Verification items for the finished model (mm, model axes). Face numbers are marked on the shaded views. A direction names the side the tool comes from. Give positions to 0.01 mm unless a question says otherwise; leave off trailing zeros. Loops run counter-clockwise (first coordinate to the right, second up) from the corner with the lowest first, then second, coordinate; pieces in that order, holes last. Notation, with made-up numbers: M 46,21.5 L 59,21.5 A24 ccw 59,33.5 Z; hole C -13.5,-4 d10. An arc over 180 degrees is marked long. Use CSV: the item, a comma, the result in double quotes.
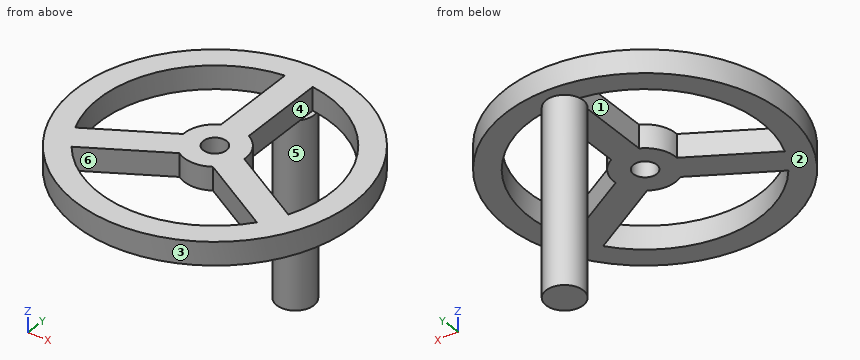
from build123d import *

# Parameters (mm, degrees)
SKETCH1_R           = 76.2
SKETCH1_R_2         = 63.5
SKETCH1_R_3         = 16.816105372
SKETCH1_R_4         = 6.35
BOSS_EXTRUDE1_DEPTH = 12.7
SKETCH2_R           = 10.16
BOSS_EXTRUDE2_DEPTH = 101.6


with BuildPart() as part:
    # Sketch1 → Boss-Extrude1 (new body)
    # profile 1 of 6: a face of its own
    with BuildSketch(Plane.XY):
        Circle(SKETCH1_R)
        Circle(SKETCH1_R_2, mode=Mode.SUBTRACT)
    # profile 2 of 6: a face of its own
    with BuildSketch(Plane.XY):
        with BuildLine():
            ThreePointArc((-7.62, 14.990563695), (-3.917811966, 16.353352845), (0, 16.816105372))
            Line((0, 16.816105372), (0, 63.5))
            ThreePointArc((0, 63.5), (-3.816901576, 63.385181725), (-7.62, 63.041142122))
            Line((-7.62, 63.041142122), (-7.62, 14.990563695))
        make_face()
    # profile 3 of 6: a face of its own
    with BuildSketch(Plane.XY):
        with BuildLine():
            Line((0, 63.5), (0, 16.816105372))
            ThreePointArc((0, 16.816105372), (3.917811966, 16.353352845), (7.62, 14.990563695))
            Line((7.62, 14.990563695), (7.62, 63.041142122))
            ThreePointArc((7.62, 63.041142122), (3.816901576, 63.385181725), (0, 63.5))
        make_face()
    # profile 4 of 6: a face of its own
    with BuildSketch(Plane.XY):
        with BuildLine():
            ThreePointArc((-9.172208976, -14.094395424), (-14.563174445, -8.408052686), (-16.792208976, -0.89616827))
            Line((-16.792208976, -0.89616827), (-58.405230561, -24.921457484))
            ThreePointArc((-58.405230561, -24.921457484), (-54.99261314, -31.75), (-50.785230561, -38.119684638))
            Line((-50.785230561, -38.119684638), (-9.172208976, -14.094395424))
        make_face()
    # profile 5 of 6: a face of its own
    with BuildSketch(Plane.XY):
        with BuildLine():
            Line((58.405230561, -24.921457484), (16.792208976, -0.89616827))
            ThreePointArc((16.792208976, -0.89616827), (14.563174445, -8.408052686), (9.172208976, -14.094395424))
            Line((9.172208976, -14.094395424), (50.785230561, -38.119684638))
            ThreePointArc((50.785230561, -38.119684638), (54.99261314, -31.75), (58.405230561, -24.921457484))
        make_face()
    # profile 6 of 6: a face of its own
    with BuildSketch(Plane.XY):
        Circle(SKETCH1_R_3)
        Circle(SKETCH1_R_4, mode=Mode.SUBTRACT)
    extrude(amount=BOSS_EXTRUDE1_DEPTH)

    # Sketch2 → Boss-Extrude2 (add)
    with BuildSketch(Plane(origin=(0, 0, 0), x_dir=(-1, 0, 0), z_dir=(0, 0, -1))):
        with Locations(Location((0, 60.427828817, 0), (0, 0, 166.938408153))):
            Circle(SKETCH2_R)
    extrude(amount=BOSS_EXTRUDE2_DEPTH)


solid = part.part
(1) Section check A-A on x = 0. Record the cut outline in (y, z), plus the area to 3 significant figures.
Calculated:
outline,"M -76.2,0 L -63.5,0 L -63.5,12.7 L -76.2,12.7 Z; M -16.82,0 L -6.35,0 L -6.35,12.7 L -16.82,12.7 Z; M 6.35,0 L 50.27,0 L 50.27,-101.6 L 70.59,-101.6 L 70.59,0 L 76.2,0 L 76.2,12.7 L 6.35,12.7 Z"
area,"3,250 mm²"
(2) Scan lines: L1, parallel to X at y = -7, z = 1; L2, parallel to Z at x = 50, y = -27.5; L3, parallel to X at y = -47, z = 3. Record each from-to range of solid material in increasing order. Write a range as from..to.
Calculated:
L1,"x = -75.88..-63.11, -27.36..27.36, 63.11..75.88"
L2,"z = 0..12.7"
L3,"x = -59.98..-42.7, 42.7..59.98"
(3) Mould release check, pull along Y, two halves, no side actions. Record for the marked faces 1, 2 and 3: released by +Y, released by -Y, zero draft, split by the parting line, or undercut.
Calculated:
face 1,"undercut"
face 2,"zero draft"
face 3,"split by the parting line"
(4) Section check B-B on y = -58.5. Record the cut outline in (x, z).
Calculated:
outline,"M -48.83,0 L -24.7,0 L -24.7,12.7 L -48.83,12.7 Z; M 24.7,0 L 48.83,0 L 48.83,12.7 L 24.7,12.7 Z"
(5) Section check D-D on x = 19. Record the cut outline in (y, z).
Calculated:
outline,"M -73.79,0 L -60.59,0 L -60.59,12.7 L -73.79,12.7 Z; M -19.77,0 L -2.17,0 L -2.17,12.7 L -19.77,12.7 Z; M 60.59,0 L 73.79,0 L 73.79,12.7 L 60.59,12.7 Z"
(6) Section check C-C on y = 42. Record the cut outline in (x, z), plus the area to 3 significant figures.
Calculated:
outline,"M -63.58,0 L -47.63,0 L -47.63,12.7 L -63.58,12.7 Z; M -7.62,0 L 7.62,0 L 7.62,12.7 L -7.62,12.7 Z; M 47.63,0 L 63.58,0 L 63.58,12.7 L 47.63,12.7 Z"
area,"599 mm²"
(7) Tool access check on the marked faces 4, 5 and 6. Record the directions out of +Z, -Z, +X, -X, +Y, -Y that give a thin tool (end or side, any length) a straight path to the whole face; none if there is none.
Calculated:
face 4,"+Z"
face 5,"-Z"
face 6,"+Z, -Z"
(8) Depth check by flat-ended pin: pin 1 Ø10 at (y, z) = (40, 6) entering from -X; pin 2 Ø10 at (x, y) = (-54.5, 50) entering from -Z; pin 3 Ø0.8 at (x, y) = (9, 59.5) entering from +Z. Enter the tip coordinate at first touch or a pass-through.
Calculated:
pin 1,"stops at x = -67.69"
pin 2,"stops at z = 0"
pin 3,"stops at z = 0"
